```python
from build123d import *

# Parameters (mm, degrees)
SKETCH1_W           = 645.16
SKETCH1_H           = 645.16
BOSS_EXTRUDE1_DEPTH = 190.5
CHAMFER1_SIZE       = 127
SKETCH2_R           = 152.4
CUT_EXTRUDE1_DEPTH  = 595.370854602
SKETCH3_R           = 152.4
CUT_EXTRUDE2_DEPTH  = 747.042580554
CIRPATTERN1_COUNT   = 4


with BuildPart() as part:
    # Sketch1 → Boss-Extrude1 (new, symmetric)
    with BuildSketch(Plane(origin=(0, 0, 0), x_dir=(1, 0, 0), z_dir=(0, 1, 0))):
        Rectangle(SKETCH1_W, SKETCH1_H)
    extrude(amount=BOSS_EXTRUDE1_DEPTH, both=True)

    # Chamfer1
    chamfer1_edges = [part.edges().sort_by_distance(p)[0] for p in [
        (322.58, 0, 322.58),
        (-322.58, 0, 322.58),
        (-322.58, 0, -322.58),
        (322.58, 0, -322.58),
    ]]
    chamfer(chamfer1_edges, length=CHAMFER1_SIZE)

    # Sketch2 → Cut-Extrude1 (cut, through all)
    with BuildSketch(Plane(origin=(0, 190.5, 0), x_dir=(1, 0, 0), z_dir=(0, 1, 0))):
        with Locations(Location((0, 0, 0), (0, 0, 270))):
            Circle(SKETCH2_R)
    extrude(amount=-CUT_EXTRUDE1_DEPTH, mode=Mode.SUBTRACT)

    # Sketch3 → Cut-Extrude2 (cut, through all)
    with BuildSketch(Plane.XY.offset(322.58)):
        Circle(SKETCH3_R)
    cut_extrude2 = extrude(amount=-CUT_EXTRUDE2_DEPTH, mode=Mode.SUBTRACT)

    # CirPattern1: Cut-Extrude2 ×4 about axis
    cirpattern1_axis = Axis((0, -190.5, 0), (0, 1, 0))
    for i in range(1, CIRPATTERN1_COUNT):
        add(cut_extrude2.rotate(cirpattern1_axis, i * 360 / CIRPATTERN1_COUNT), mode=Mode.SUBTRACT)


solid = part.part
```
Geometry: final body of the model. Coordinates: model frame, mm. Coordinates: 2 decimals unless noted, no trailing zeros. Order: outer loops, then holes, each group sorted by start corner. A loop starts at its lowest first (then second) coordinate and runs counter-clockwise, first axis right, second up. Notation, with made-up numbers: (80.25, 73) - (115.25, 73) arc R7 ccw to (115.25, 78) - close; hole circle Ø10 at (36, -25.75). An arc over 180 degrees is marked (long way). Write each question's results on one line, items separated by ' | '.
1) Section A-A, the plane y = 0. Return loops of the section in (x, z).
Results list:
outline: (-322.58, -195.58) - (-195.58, -322.58) - (-152.4, -322.58) - (-152.4, -152.4) - (-322.58, -152.4) - close; (-322.58, 152.4) - (-152.4, 152.4) - (-152.4, 322.58) - (-195.58, 322.58) - (-322.58, 195.58) - close; (152.4, -322.58) - (195.58, -322.58) - (322.58, -195.58) - (322.58, -152.4) - (152.4, -152.4) - close; (152.4, 152.4) - (322.58, 152.4) - (322.58, 195.58) - (195.58, 322.58) - (152.4, 322.58) - close
2) Section B-B, the plane z = 0. Return loops of the section in (x, y).
Results list:
outline: (-322.58, -190.5) - (-152.4, -190.5) - (-152.4, -152.4) - (-322.58, -152.4) - close; (-322.58, 152.4) - (-152.4, 152.4) - (-152.4, 190.5) - (-322.58, 190.5) - close; (152.4, -190.5) - (322.58, -190.5) - (322.58, -152.4) - (152.4, -152.4) - close; (152.4, 152.4) - (322.58, 152.4) - (322.58, 190.5) - (152.4, 190.5) - close
3) Section D-D, the plane z = -239.5. Return loops of the section in (x, y), plus the area to 3 significant figures.
Results list:
outline: (-278.66, -190.5) - (278.66, -190.5) - (278.66, 190.5) - (-278.66, 190.5) - close; hole circle Ø304.8 at (0, 0) | area: 139,000 mm^2
4) Line query: line 1 (Y direction, x = 0, z = 193); line 2 (X direction, y = -169.5, z = 0). Output: solid intervals per line, ascending. Write a range as from..to.
Results list:
line 1: -190.5..-152.4, 152.4..190.5 | line 2: -322.58..-152.4, 152.4..322.58
5) Section C-C, the plane x = 53.5. Return loops of the section in (y, z), plus the area to 3 significant figures.
Results list:
outline: (-190.5, -322.58) - (-142.7, -322.58) - (-142.7, -142.7) - (-190.5, -142.7) - close; (-190.5, 142.7) - (-142.7, 142.7) - (-142.7, 322.58) - (-190.5, 322.58) - close; (142.7, -322.58) - (190.5, -322.58) - (190.5, -142.7) - (142.7, -142.7) - close; (142.7, 142.7) - (190.5, 142.7) - (190.5, 322.58) - (142.7, 322.58) - close | area: 34,400 mm^2
6) Pull-direction query (X, two-part tool) for faces 1 (the cylindrical face through (6.701, 158.904, -152.253)), 2 (the cylindrical face through (-112.325, 102.999, -237.536)), 3 (the flat face through (-90, 130, -322.58)), 4 (the flat face through (322.58, 130, 90)); classes: pulls with the +X half, pulls with the -X half, needs draft (parallel to the pull), parting line crosses it, or undercut.
Results list:
face 1: undercut | face 2: undercut | face 3: needs draft | face 4: pulls with the +X half
